Autodesk Inventor part; units mm, degrees
ref_plane "YZ Plane" through (0, 0, 0) normal (1, 0, 0) x (0, 1, 0)
ref_plane "XZ Plane" through (0, 0, 0) normal (0, 1, 0) x (-1, 0, 0)
ref_plane "XY Plane" through (0, 0, 0) normal (0, 0, 1) x (1, 0, 0)
sketch "Sketch1" plane through (0, 0, 0) normal (0, 0, 1) x (1, 0, 0)
  line L0 (52.418, 170.3116) -> (67.15, 170.3116)
  line L1 (67.15, 170.3116) -> (67.15, 167.2636)
  line L2 (51.148, 171.5816) -> (51.148, 186.3136)
  line L3 (51.148, 186.3136) -> (52.926, 186.3136)
  line L4 (54.196, 185.0436) -> (54.196, 173.3596)
  line L5 (67.15, 170.3116) -> (67.15, 172.0896)
  line L6 (65.88, 173.3596) -> (54.196, 173.3596)
  arc A0 (54.196, 185.0436) -> (52.926, 186.3136) centre (52.926, 185.0436) ccw
  arc A1 (67.15, 172.0896) -> (65.88, 173.3596) centre (65.88, 172.0896) ccw
  arc A2 (51.148, 171.5816) -> (52.418, 170.3116) centre (52.418, 171.5816) ccw
  point P0 (0, 0)
  point P1 (51.148, 170.3116)
  point P2 (54.196, 186.3136)
  point P3 (67.15, 173.3596)
  dimension "d0" = 16.002
  dimension "d1" = 3.048
  dimension "d2" = 16.002
  dimension "d3" = 3.048
  dimension "d4" = 3.048
  dimension "d5" = 1.27
  dimension "d6" = 1.27
extrude "Extrusion1" add sketch "Sketch1" along normal blind 146.304
sketch "Sketch3" plane through (54.196, 173.3596, 0) normal (0, 1, 0) x (1, 0, 0)
  line L0 (0.9375, 6.2475) -> (13.2819, 6.2475)
  line L1 (12.954, 0) -> (-1.778, 0)
  line L2 (5.588, 0) -> (5.588, -6.1341)
  line L3 (-1.778, -146.304) -> (12.954, -146.304)
  circle A0 centre (5.588, -7.9756) radius 1.8415
  line L4 (5.588, -7.9756) -> (5.588, -130.5306)
  circle A1 centre (5.588, -134.2136) radius 1.8415
  point P0 (-54.196, 0)
  dimension "d31" = 12.3444
  dimension "d32" = 6.1341
  dimension "d38" = 122.555
extrude "Extrusion6" cut sketch "Sketch3" against normal blind 69.85
sketch "Sketch4" plane through (54.196, 173.3596, 0) normal (0, 1, 0) x (1, 0, 0)
  circle A0 centre (5.588, -7.9756) radius 1.8415
  line L0 (5.588, -25.6184) -> (6.1855, -25.6184)
  circle A1 centre (5.588, -23.7769) radius 1.8415
  circle A2 centre (5.588, -39.5757) radius 1.8415
  circle A3 centre (5.588, -55.3745) radius 1.8415
  circle A4 centre (5.588, -71.1733) radius 1.8415
  circle A5 centre (5.588, -86.9721) radius 1.8415
  circle A6 centre (5.588, -102.7709) radius 1.8415
  circle A7 centre (5.588, -118.5697) radius 1.8415
  point P0 (-54.196, 0)
extrude "Extrusion7" cut sketch "Sketch4" against normal blind 34.925 contours A1 | A2 | A3 | A4 | A5 | A6 | A7
properties part number "L Bracket with holes"
Part model, mm, in its own coordinate system. A direction names the side the tool comes from. Coordinates: 2 decimals unless noted, no trailing zeros. Order: outer loops, then holes, each group sorted by start corner. A loop starts at its lowest first (then second) coordinate and runs counter-clockwise, first axis right, second up. Notation, with made-up numbers: (31.5, -33) - (49.5, -33) arc R20 cw to (49.5, -15) - close; hole circle Ø4 at (-25, -15). An arc over 180 degrees is marked (long way). Use CSV: the item, a comma, the result in double quotes.
Item 1: Saw through at A-A on z = 13. Give the cut face in (x, y), and give its area (3 significant figures).
Solved:
outline,"(51.15, 171.58) arc R1.27 ccw to (52.42, 170.31) - (67.15, 170.31) - (67.15, 172.09) arc R1.27 ccw to (65.88, 173.36) - (54.2, 173.36) - (54.2, 185.04) arc R1.27 ccw to (52.93, 186.31) - (51.15, 186.31) - close"
area,"87.2 mm²"
Item 2: Mould opens along Z. For faces 1 (the face through (59.54, 171.86, 132.39)), 2 (the face through (54, 175, 146.304)), 3 (the face through (57.944, 171.857, 23.696)), 4 (the face through (58, 170.312, 72.1)) say: +Z half, -Z half, draft (parallel to the pull), parting line (faces both ways), or undercut.
Solved:
face 1,"undercut"
face 2,"+Z half"
face 3,"undercut"
face 4,"draft"
Item 3: Probe probe 1 along Y at (x, z) = (56.5, 40); probe 2 along X at (y, z) = (179, 69); probe 3 along X at (y, z) = (172, 57). List the from-to ranges inside material, lowest first.
Solved:
probe 1,"y = 170.31 to 173.36"
probe 2,"x = 51.15 to 54.2"
probe 3,"x = 51.15 to 58.92, 60.65 to 67.15"
Item 4: Saw through at B-B on y = 177. Give the cut face in (x, z), and give its area (3 significant figures).
Solved:
outline,"(51.15, 0) - (54.2, 0) - (54.2, 146.3) - (51.15, 146.3) - close"
area,"446 mm²"
Item 5: 3-axis set-ups, long thin cutter, end or side, ignore diameter. For faces 5 (the face through (54.196, 179, 72)), 6 (the face through (59.54, 171.86, 53.55)): which of +Z, -Z, +X, -X, +Y, -Y reach the whole face in a straight line?
Solved:
face 5,"+Z, -Z, +X, +Y"
face 6,"+Y, -Y"
Item 6: Drop flat-ended pins along their axis: P1, Ø3, axis at x = 59.78, z = 7.98, coming from the -Y side; P2, Ø3.5, axis at x = 59, z = 62, coming from the +Y side; P3, Ø3.5, axis at y = 182, z = 45, coming from the +X side. Give the stop position or say it passes through.
Solved:
P1,"passes through"
P2,"stops at y = 173.36"
P3,"stops at x = 54.2"
Item 7: Saw through at C-C on x = 63.75. Give the cut face in (y, z).
Solved:
outline,"(170.31, 0) - (173.36, 0) - (173.36, 146.3) - (170.31, 146.3) - close"
